Build history of the part. All positions in model axes, mm. Give positions to 0.01 mm unless a question says otherwise; leave off trailing zeros. Loops run counter-clockwise (first coordinate to the right, second up) from the corner with the lowest first, then second, coordinate; pieces in that order, holes last. Notation, with made-up numbers: (26, 5.5) - (36, 5.5) arc R37 cw to (36, 42.5) - close; hole circle Ø10 at (23, 54). An arc over 180 degrees is marked (long way). Return JSON: item names as keys, results as strings. Group by question number.
1) Drill centre lines: probe 1 along X at (y, z) = (6.25, 3.5); probe 2 along Z at (x, y) = (4.75, 2.5); probe 3 along X at (y, z) = (6, -0.75). Where is each one in solid material? Low to high. Write a range as from..to.
2) Slice it at A-A (z = 3.5). List the corners of the cut face in (x, y).
3) Slice it at B-B (y = 5.75). List the corners of the cut face in (x, z), and give its area (3 significant figures).
4) Drop a flat-ended pin along its axis: pin 1 (3 mm diameter, centred on x = -5, z = 3.5, fed in from +Y). Give the stop position or say it passes through.
5) Mould opens along X. For faces 1 (the face through (-9.5, 4, 4)), 2 (the face through (6.644, 4.056, 4.548)), 3 (the face through (9.5, 4, 4)), 4 (the face through (-6.73, 4.06, 4.4)) say: released by +X, released by -X, zero draft, split by the parting line, or undercut.
6) Slice it at D-D (z = 2.5). List the corners of the cut face in (x, y), and give its area (3 significant figures).
7) Slice it at C-C (x = 5). List the corners of the cut face in (y, z), and give its area (3 significant figures).
```python
from build123d import *

# Parameters (mm, degrees)
SKETCH_1_W           = 30
SKETCH_1_H           = 15
EXTRUDE_1_DEPTH      = 8
FILLET_1_R           = 6
SKETCH_2_R           = 1.95
CUT_EXTRUDE_1_DEPTH  = 19.580904176
SKETCH_3_OUTSIDE_W   = 38.896
SKETCH_3_OUTSIDE_H   = 23.896
SKETCH_3_OUTSIDE_W_2 = 19
SKETCH_3_OUTSIDE_H_2 = 10
CUT_EXTRUDE_3_DEPTH  = 10
FILLET_3_R           = 2


with BuildPart() as part:
    # Эскиз1 → Бобышка-Вытянуть1 (new body)
    with BuildSketch(Plane(origin=(0, 0, 0), x_dir=(1, 0, 0), z_dir=(0, 1, 0))):
        Rectangle(SKETCH_1_W, SKETCH_1_H)
    extrude(amount=EXTRUDE_1_DEPTH)

    # Скругление1
    fillet_1_edges = [part.edges().sort_by_distance(p)[0] for p in [
        (-15, 4, -7.5),
        (15, 4, -7.5),
    ]]
    fillet(fillet_1_edges, radius=FILLET_1_R)

    # Эскиз2 → Вырез-Вытянуть1 (cut, through all)
    with BuildSketch(Plane(origin=(0, 8, 0), x_dir=(1, 0, 0), z_dir=(0, 1, 0))):
        with Locations(Location((-5, -3.5, 0), (0, 0, 270))):
            Circle(SKETCH_2_R)
        with Locations(Location((5, -3.5, 0), (0, 0, 270))):
            Circle(SKETCH_2_R)
    extrude(amount=-CUT_EXTRUDE_1_DEPTH, mode=Mode.SUBTRACT)

    # Эскиз3 outside → Вырез-Вытянуть3 (cut)
    with BuildSketch(Plane(origin=(0, 8, 0), x_dir=(1, 0, 0), z_dir=(0, 1, 0))):
        Rectangle(SKETCH_3_OUTSIDE_W, SKETCH_3_OUTSIDE_H)
        with Locations((0, -2.5)):
            Rectangle(SKETCH_3_OUTSIDE_W_2, SKETCH_3_OUTSIDE_H_2, mode=Mode.SUBTRACT)
    extrude(amount=-CUT_EXTRUDE_3_DEPTH, mode=Mode.SUBTRACT)

    # Скругление3
    fillet_3_edges = [part.edges().sort_by_distance(p)[0] for p in [
        (-9.5, 4, -2.5),
        (9.5, 4, -2.5),
    ]]
    fillet(fillet_3_edges, radius=FILLET_3_R)


solid = part.part
```
Results:
{
 "1": {"probe 1": "-9.5..-6.95, -3.05..3.05, 6.95..9.5", "probe 2": "-2.5..1.57, 5.43..7.5", "probe 3": "-9.48..9.48"},
 "2": {"outline": "(-9.5, 0) - (-6.95, 0) - (-6.95, 8) - (-9.5, 8) - close; (-3.05, 0) - (3.05, 0) - (3.05, 8) - (-3.05, 8) - close; (6.95, 0) - (9.5, 0) - (9.5, 8) - (6.95, 8) - close"},
 "3": {"outline": "(-9.5, -0.5) arc R2 ccw to (-7.5, -2.5) - (7.5, -2.5) arc R2 ccw to (9.5, -0.5) - (9.5, 7.5) - (-9.5, 7.5) - close; hole circle Ø3.9 at (-5, 3.5); hole circle Ø3.9 at (5, 3.5)", "area": "164 mm2"},
 "4": {"pin 1": "through"},
 "5": {"face 1": "released by -X", "face 2": "undercut", "face 3": "released by +X", "face 4": "undercut"},
 "6": {"outline": "(-9.5, 0) - (-6.67, 0) - (-6.67, 8) - (-9.5, 8) - close; (-3.33, 0) - (3.33, 0) - (3.33, 8) - (-3.33, 8) - close; (6.67, 0) - (9.5, 0) - (9.5, 8) - (6.67, 8) - close", "area": "98.4 mm2"},
 "7": {"outline": "(0, -2.5) - (8, -2.5) - (8, 1.55) - (0, 1.55) - close; (0, 5.45) - (8, 5.45) - (8, 7.5) - (0, 7.5) - close", "area": "48.8 mm2"}
}
